Geometry check sheet. Reference: the model listing, model coordinates, mm. Face numbers are marked on the shaded views. A direction names the side the tool comes from. Coordinates: 2 decimals unless noted, no trailing zeros. Order: outer loops, then holes, each group sorted by start corner. A loop starts at its lowest first (then second) coordinate and runs counter-clockwise, first axis right, second up. Notation, with made-up numbers: (64, 67) - (86, 67) arc R17 cw to (86, 83) - close; hole circle Ø6 at (30.5, 77.5). An arc over 180 degrees is marked (long way). Return JSON: item names as keys, results as strings. Group by question number.
Item 1: Scan lines: probe 1 along X at (y, z) = (63.5, 15); probe 2 along Z at (x, y) = (58, 59) (3 decimals); probe 3 along Y at (x, z) = (87.5, 8.5). Record each from-to range of solid material in increasing order.
Item 2: Section check D-D on z = -19. Enter the section's corners in (x, y) (3 decimals), then the cut area to 3 significant figures.
Item 3: Gauge pin test, flat ends, axial feed: pin 1 (8 mm diameter, centred on x = -24.5, y = 106, fed in from -Z); pin 2 (19 mm diameter, centred on x = -16, z = -9, fed in from +Y); pin 3 (3.5 mm diameter, centred on y = 90, z = 2, fed in from +X). Record the tip position at first contact, or that the pin passes through.
Item 4: Tool access check on the marked faces 4 and 5. Record the directions out of +Z, -Z, +X, -X, +Y, -Y that give a thin tool (end or side, any length) a straight path to the whole face; none if there is none.
Item 5: Draft check along X on the marked faces 1, 2 and 3. Enter one of: pulls with the +X half, pulls with the -X half, needs draft (parallel to the pull), parting line crosses it, or undercut.
Item 6: Section check A-A on z = -10. Enter the section's corners in (x, y) (3 decimals).
Item 7: Section check C-C on x = 32. Enter the section's corners in (y, z) (3 decimals), then the cut area to 3 significant figures.
Item 8: Section check B-B on y = 76.5. Enter the section's corners in (x, z) (3 decimals), then the cut area to 3 significant figures.
from build123d import *

# Parameters (mm, degrees)
SKETCH1_W               = 203.2
SKETCH1_H               = 63.5
BOSS_EXTRUDE1_DEPTH     = 101.6
SKETCH3_W               = 190.5
SKETCH3_H               = 11.43
CUT_EXTRUDE1_DEPTH      = 6.35
CUT_EXTRUDE2_DEPTH      = 11.43
SKETCH5_R               = 6.35
BOSS_EXTRUDE2_DEPTH     = 19.05
CUT_EXTRUDE3_DEPTH      = 163.119118937
CUT_EXTRUDE3_DEPTH_BACK = 163.119118937
SKETCH6_R               = 1.125000036


with BuildPart() as part:
    # Sketch1 → Boss-Extrude1 (new body)
    with BuildSketch(Plane(origin=(0, 0, 0), x_dir=(1, 0, 0), z_dir=(0, 1, 0))):
        Rectangle(SKETCH1_W, SKETCH1_H)
    extrude(amount=BOSS_EXTRUDE1_DEPTH)

    # Sketch3 → Cut-Extrude1 (cut)
    with BuildSketch(Plane(origin=(0, 101.6, 0), x_dir=(1, 0, 0), z_dir=(0, 1, 0))):
        with Locations((6.35, 0)):
            Rectangle(SKETCH3_W, SKETCH3_H)
    extrude(amount=-CUT_EXTRUDE1_DEPTH, mode=Mode.SUBTRACT)

    # Sketch4 → Cut-Extrude2 (cut)
    with BuildSketch(Plane.XY.offset(-5.715)):
        Polygon((-88.9, 101.6), (-88.9, 57.15), (101.6, 12.7), (101.6, 101.6), align=None)
    extrude(amount=CUT_EXTRUDE2_DEPTH, mode=Mode.SUBTRACT)

    # Sketch5 → Boss-Extrude2 (add)
    with BuildSketch(Plane(origin=(0, 101.6, 0), x_dir=(1, 0, 0), z_dir=(0, 1, 0))):
        with Locations(Location((88.9, -18.7325, 0), (0, 0, 90))):
            Circle(SKETCH5_R)
        with Locations(Location((-88.9, -18.7325, 0), (0, 0, 90))):
            Circle(SKETCH5_R)
        with Locations(Location((-88.9, 18.7325, 0), (0, 0, 90))):
            Circle(SKETCH5_R)
        with Locations(Location((88.9, 18.7325, 0), (0, 0, 90))):
            Circle(SKETCH5_R)
    extrude(amount=BOSS_EXTRUDE2_DEPTH)

    # Sketch6 → Cut-Extrude3 (cut, two sides: drawn at the far end of the back side and taken through both)
    with BuildSketch(Plane.XY.offset(-5.715).offset(-CUT_EXTRUDE3_DEPTH_BACK)):
        with Locations((88.265, 63.5)):
            Circle(SKETCH6_R)
    extrude(amount=CUT_EXTRUDE3_DEPTH + CUT_EXTRUDE3_DEPTH_BACK, mode=Mode.SUBTRACT)


solid = part.part
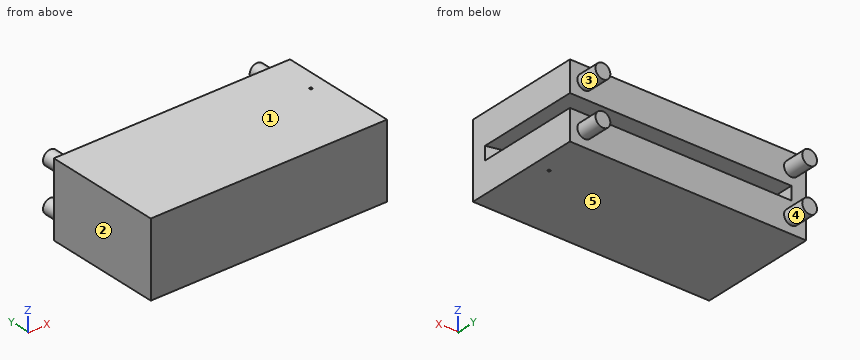
Computed:
{
 "1": {"probe 1": "x = -101.6 to 87.14, 89.39 to 101.6", "probe 2": "z = -31.75 to -5.715, 5.715 to 31.75", "probe 3": "y = 0 to 62.68, 64.32 to 101.6"},
 "2": {"outline": "(-101.6, 0) - (101.6, 0) - (101.6, 101.6) - (95.244, 101.6) - (95.244, 120.65) - (82.556, 120.65) - (82.556, 101.6) - (-82.556, 101.6) - (-82.556, 120.65) - (-95.244, 120.65) - (-95.244, 101.6) - (-101.6, 101.6) - close; hole circle Ø2.25 at (88.265, 63.5)", "area": "21,100 mm²"},
 "3": {"pin 1": "passes through", "pin 2": "stops at y = 101.6", "pin 3": "stops at x = -88.9"},
 "4": {"face 4": "+Y", "face 5": "-Z, +X, -X, +Y, -Y"},
 "5": {"face 1": "needs draft", "face 2": "pulls with the -X half", "face 3": "undercut"},
 "6": {"outline": "(-101.6, 0) - (101.6, 0) - (101.6, 101.6) - (-101.6, 101.6) - close; hole circle Ø2.25 at (88.265, 63.5)"},
 "7": {"outline": "(0, -31.75) - (101.6, -31.75) - (101.6, -5.715) - (28.94, -5.715) - (28.94, 5.715) - (101.6, 5.715) - (101.6, 31.75) - (0, 31.75) - close", "area": "5,620 mm²"},
 "8": {"outline": "(-101.6, -31.75) - (101.6, -31.75) - (101.6, -5.715) - (-88.9, -5.715) - (-88.9, 5.715) - (101.6, 5.715) - (101.6, 31.75) - (-101.6, 31.75) - close", "area": "10,700 mm²"}
}
